Input: part model. Units: mm. Frame: model coordinates. Face numbers are marked on the shaded views. A direction names the side the tool comes from. Round coordinates to 2 decimals unless told otherwise and drop trailing zeros. Loops run counter-clockwise (first coordinate to the right, second up) from the corner with the lowest first, then second, coordinate; pieces in that order, holes last. Notation, with made-up numbers: (81.25, -26.5) - (125.25, -26.5) arc R10 ccw to (125.25, -9.5) - close; hole circle Ø8 at (1.5, -29.5). An arc over 180 degrees is marked (long way). Write each question's results on one line, items separated by ' | '.
Autodesk Fusion 360 part; units mm, degrees
sketch "Esquisse1" plane through (0, 0, 0) normal (0, 0, 1) x (1, 0, 0)
  line L0 (0, 0) -> (300, 0)
  line L1 (300, 0) -> (300, 150)
  line L2 (300, 150) -> (0, 150)
  line L3 (0, 150) -> (0, 0)
extrude "Extrusion1" add sketch "Esquisse1" along normal blind 75
chamfer "Chanfrein1" distance 30 angle 45 1 edges at (150, 0, 75)
chamfer "Chanfrein2" distance 30 angle 45 1 edges at (150, 150, 75)
box "BoitePrimitive1" add length 50 width 50 height 25 placed x (0, -1, 0) y (1, 0, 0) z (0, 0, 1) at (125, 100, 75)
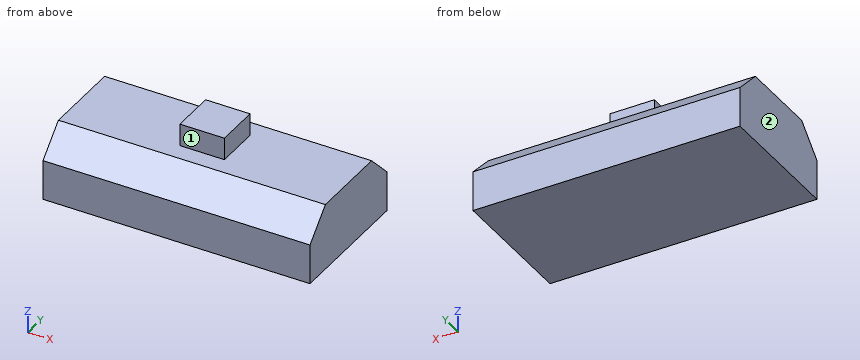
1. Section query D-D, the plane x = 208. Output: boundary loops of the cut face in (y, z), plus the area to 4 significant figures.
Answer:
outline: (0, 0) - (150, 0) - (150, 45) - (120, 75) - (30, 75) - (0, 45) - close | area: 10,350 mm^2
2. Contact query for flat-ended pins moving along their axis: pin 1 (12.5 mm diameter, centred on x = 153.5, z = 84, fed in from -Y); pin 2 (10 mm diameter, centred on y = 65.5, z = 61.5, fed in from -X); pin 3 (12 mm diameter, centred on x = 188, y = 109.5, fed in from +Z); pin 4 (12.5 mm diameter, centred on x = 151, z = 89, fed in from +Y). Output: stop coordinate, or through.
Answer:
pin 1: y = 50 | pin 2: x = 0 | pin 3: z = 75 | pin 4: y = 100
3. Section query C-C, the plane z = 61.5. Output: boundary loops of the cut face in (x, y).
Answer:
outline: (0, 16.5) - (300, 16.5) - (300, 133.5) - (0, 133.5) - close
4. Line query: line 1 (Z direction, x = 20, y = 93); line 2 (Y direction, x = 224.5, z = 53.5); line 3 (Y direction, x = 153.5, z = 92.5). Output: solid intervals per line, ascending. Write a range as [from, to].
Answer:
line 1: [0, 75] | line 2: [8.5, 141.5] | line 3: [50, 100]
5. Set-up query: the marked faces 1 and 2. Return all of +Z, -Z, +X, -X, +Y, -Y with unobstructed straight access to the full face (end or side cutting, diameter ignored); none if empty.
Answer:
face 1: +Z, +X, -X, -Y | face 2: +Z, -Z, -X, +Y, -Y
6. Section query A-A, the plane y = 76.5. Output: boundary loops of the cut face in (x, z), plus the area to 4 significant figures.
Answer:
outline: (0, 0) - (300, 0) - (300, 75) - (175, 75) - (175, 100) - (125, 100) - (125, 75) - (0, 75) - close | area: 23,750 mm^2
7. Section query B-B, the plane x = 153. Output: boundary loops of the cut face in (y, z), plus the area to 3 significant figures.
Answer:
outline: (0, 0) - (150, 0) - (150, 45) - (120, 75) - (100, 75) - (100, 100) - (50, 100) - (50, 75) - (30, 75) - (0, 45) - close | area: 11,600 mm^2
